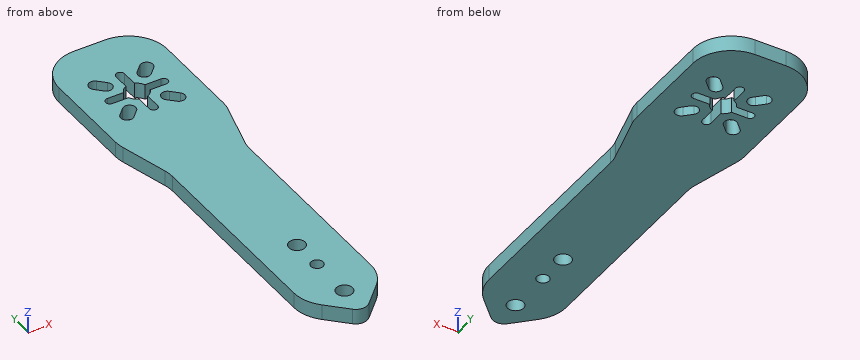
```python
from build123d import *

# Parameters (mm, degrees)
F0_R     = 2.1
F0_R_2   = 1.6
F1_DEPTH = 4
F2_R     = 10
F3_R     = 3


with BuildPart() as f1:
    # F0 (on Top) → F1 (new body)
    with BuildSketch(Plane.XY):
        Polygon((-10, 67.571797), (-10, 11), (0, 1), (10, 11), (10, 67.571797), (14, 82.5), (14, 117.5), (-14, 117.5), (-14, 82.5), align=None)
        with Locations((0, 10)):
            Circle(F0_R, mode=Mode.SUBTRACT)
        with Locations((0, 21.566757)):
            Circle(F0_R_2, mode=Mode.SUBTRACT)
        with Locations((0, 30)):
            Circle(F0_R, mode=Mode.SUBTRACT)
        with BuildLine():
            ThreePointArc((-5.586144, 89.651115), (-7.848885, 89.651115), (-7.848885, 91.913856))
            Line((-7.848885, 91.913856), (-6.081118, 93.681623))
            ThreePointArc((-6.081118, 93.681623), (-3.818377, 93.681623), (-3.818377, 91.418882))
            Line((-3.818377, 91.418882), (-5.586144, 89.651115))
        make_face(mode=Mode.SUBTRACT)
        with BuildLine():
            ThreePointArc((-7.848885, 103.086144), (-7.848885, 105.348885), (-5.586144, 105.348885))
            Line((-5.586144, 105.348885), (-3.818377, 103.581118))
            ThreePointArc((-3.818377, 103.581118), (-3.818377, 101.318377), (-6.081118, 101.318377))
            Line((-6.081118, 101.318377), (-7.848885, 103.086144))
        make_face(mode=Mode.SUBTRACT)
        with BuildLine():
            ThreePointArc((1.1, 100.291057), (2.12132, 99.62132), (2.791057, 98.6))
            Line((2.791057, 98.6), (7, 98.6))
            ThreePointArc((7, 98.6), (8.1, 97.5), (7, 96.4))
            Line((7, 96.4), (2.791057, 96.4))
            ThreePointArc((2.791057, 96.4), (2.12132, 95.37868), (1.1, 94.708943))
            Line((1.1, 94.708943), (1.1, 90.5))
            ThreePointArc((1.1, 90.5), (0, 89.4), (-1.1, 90.5))
            Line((-1.1, 90.5), (-1.1, 94.708943))
            ThreePointArc((-1.1, 94.708943), (-2.12132, 95.37868), (-2.791057, 96.4))
            Line((-2.791057, 96.4), (-7, 96.4))
            ThreePointArc((-7, 96.4), (-8.1, 97.5), (-7, 98.6))
            Line((-7, 98.6), (-2.791057, 98.6))
            ThreePointArc((-2.791057, 98.6), (-2.12132, 99.62132), (-1.1, 100.291057))
            Line((-1.1, 100.291057), (-1.1, 104.5))
            ThreePointArc((-1.1, 104.5), (0, 105.6), (1.1, 104.5))
            Line((1.1, 104.5), (1.1, 100.291057))
        make_face(mode=Mode.SUBTRACT)
        with BuildLine():
            ThreePointArc((7.848885, 91.913856), (7.848885, 89.651115), (5.586144, 89.651115))
            Line((5.586144, 89.651115), (3.818377, 91.418882))
            ThreePointArc((3.818377, 91.418882), (3.818377, 93.681623), (6.081118, 93.681623))
            Line((6.081118, 93.681623), (7.848885, 91.913856))
        make_face(mode=Mode.SUBTRACT)
        with BuildLine():
            ThreePointArc((5.586144, 105.348885), (7.848885, 105.348885), (7.848885, 103.086144))
            Line((7.848885, 103.086144), (6.081118, 101.318377))
            ThreePointArc((6.081118, 101.318377), (3.818377, 101.318377), (3.818377, 103.581118))
            Line((3.818377, 103.581118), (5.586144, 105.348885))
        make_face(mode=Mode.SUBTRACT)
    extrude(amount=F1_DEPTH)

    # F2
    f2_edges = [f1.edges().sort_by_distance(p)[0] for p in [
        (-14, 82.5, 2),
        (-10, 67.571797, 2),
        (-10, 11, 2),
        (10, 11, 2),
        (10, 67.571797, 2),
        (14, 82.5, 2),
        (-14, 117.5, 2),
        (14, 117.5, 2),
    ]]
    fillet(f2_edges, radius=F2_R)

    # F3
    f3_edges = [f1.edges().sort_by_distance(p)[0] for p in [
        (0, 1, 2),
    ]]
    fillet(f3_edges, radius=F3_R)


solid = f1.part
```
Read the model definition and answer for the solid it produces. Units are mm, in the model's axes. Give positions to 0.01 mm unless a question says otherwise; leave off trailing zeros. Loops run counter-clockwise (first coordinate to the right, second up) from the corner with the lowest first, then second, coordinate; pieces in that order, holes last.
Item 1: The part is cut by section A-A (y = 97.5). Write down the section's boundary in (x, z), and give its area (3 significant figures).
Item 2: Find the intervals of material crossed by line 1 along Y through (x, z) = (0, 2.2); line 2 along Y through (x, z) = (-3, 2.05); line 3 along Y through (x, z) = (6.75, 3.75), in increasing order.
Item 3: The part is cut by section B-B (x = 0). Write down the section's boundary in (y, z).
Item 4: The part is cut by section D-D (y = 48). Write down the section's boundary in (x, z), and give its area (3 significant figures).
Item 5: The part is cut by section C-C (y = 30). Write down the section's boundary in (x, z), and give its area (3 significant figures).
Item 6: Each of these flat-tipped pins is pushed along its axis until it touches: pin 1 Ø1.2 at (y, z) = (33, 1) entering from -X; pin 2 Ø1.5 at (y, z) = (73.5, 3.5) entering from +X; pin 3 Ø4 at (x, y) = (0, 30) entering from -Z; pin 4 Ø1.2 at (x, z) = (-4, 2.5) entering from -Y. Where does it stop, or does it pass through?
Taken from the geometry:
1. outline: (-14, 0) - (-8.1, 0) - (-8.1, 4) - (-14, 4) - close; (8.1, 0) - (14, 0) - (14, 4) - (8.1, 4) - close
1. area: 47.2 mm2
2. line 1: y = 2.24 to 7.9, 12.1 to 19.97, 23.17 to 27.9, 32.1 to 89.4, 105.6 to 117.5
2. line 2: y = 4 to 96.4, 98.6 to 117.5
2. line 3: y = 7.75 to 89.18, 93.01 to 96.4, 98.6 to 101.99, 105.82 to 117.11
3. outline: (2.24, 0) - (7.9, 0) - (7.9, 4) - (2.24, 4) - close; (12.1, 0) - (19.97, 0) - (19.97, 4) - (12.1, 4) - close; (23.17, 0) - (27.9, 0) - (27.9, 4) - (23.17, 4) - close; (32.1, 0) - (89.4, 0) - (89.4, 4) - (32.1, 4) - close; (105.6, 0) - (117.5, 0) - (117.5, 4) - (105.6, 4) - close
4. outline: (-10, 0) - (10, 0) - (10, 4) - (-10, 4) - close
4. area: 80.0 mm2
5. outline: (-10, 0) - (-2.1, 0) - (-2.1, 4) - (-10, 4) - close; (2.1, 0) - (10, 0) - (10, 4) - (2.1, 4) - close
5. area: 63.2 mm2
6. pin 1: stops at x = -10
6. pin 2: stops at x = 11.79
6. pin 3: passes through
6. pin 4: stops at y = 4.4
